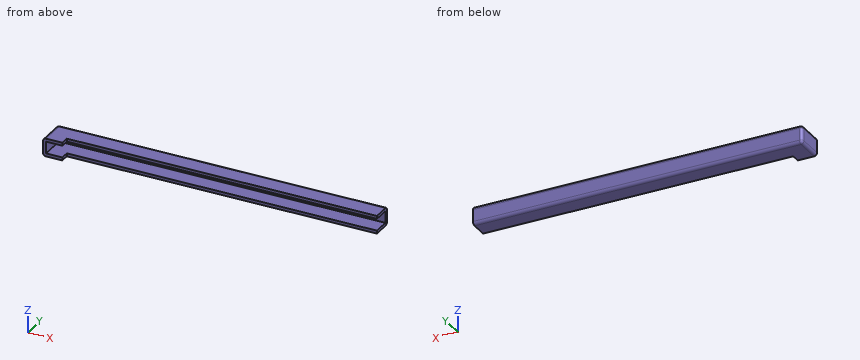
```python
from build123d import *

# Parameters (mm, degrees)
BOSS_EXTRUDE1_DEPTH = 220
SKETCH2_W           = 12
SKETCH2_H           = 13
BOSS_EXTRUDE2_DEPTH = 2
BOSS_EXTRUDE3_DEPTH = 5.8
FILLET1_R           = 2


with BuildPart() as part:
    # Sketch1 → Boss-Extrude1 (new body)
    with BuildSketch(Plane(origin=(0, 0, 0), x_dir=(0, 0, -1), z_dir=(1, 0, 0))):
        Polygon((8, 0), (8, 11), (0, 11), (0, 0), (-2, 0), (-2, 13), (10, 13), (10, 0), align=None)
    extrude(amount=BOSS_EXTRUDE1_DEPTH)

    # Sketch2 → Boss-Extrude2 (add)
    with BuildSketch(Plane.ZY):
        with Locations((-4, 6.5)):
            Rectangle(SKETCH2_W, SKETCH2_H)
    extrude(amount=BOSS_EXTRUDE2_DEPTH)

    # Sketch4 → Boss-Extrude3 (add)
    with BuildSketch(Plane.XZ):
        Polygon((0, 0), (11, 0), (11, 2), (-2, 2), (-2, -10), (11, -10), (11, -8), (0, -8), align=None)
    extrude(amount=BOSS_EXTRUDE3_DEPTH)

    # Fillet1
    fillet1_edges = [part.edges().sort_by_distance(p)[0] for p in [
        (109, 13, 2),
        (109, 13, -10),
        (-2, 3.6, -10),
        (-2, 3.6, 2),
        (-2, 13, -4),
    ]]
    fillet(fillet1_edges, radius=FILLET1_R)


solid = part.part
```
Input: part model. Units: mm. Frame: model coordinates. Coordinates: 2 decimals unless noted, no trailing zeros. Loops run counter-clockwise (first coordinate to the right, second up) from the corner with the lowest first, then second, coordinate; pieces in that order, holes last.
Q1. Section B-B, the plane y = 6.75. Return the cut outline in (x, z).
Results are:
outline: (-2, -8) arc R2 ccw to (0, -10) - (220, -10) - (220, -8) - (0, -8) - (0, 0) - (220, 0) - (220, 2) - (0, 2) arc R2 ccw to (-2, 0) - close
Q2. Section A-A, the plane z = -2.5. Return the cut outline in (x, y).
Results are:
outline: (-2, -5.8) - (0, -5.8) - (0, 11) - (220, 11) - (220, 13) - (0, 13) arc R2 ccw to (-2, 11) - close
Q3. Line query: line 1 along Z through (x, y) = (105, 10.75); line 2 along Y through (x, z) = (124, -3.5); line 3 along X through (y, z) = (0.25, -6.25). Output: solid intervals per line, ascending.
Results are:
line 1: z = -10 to -8, 0 to 2
line 2: y = 11 to 13
line 3: x = -2 to 0
Q4. Contact query for flat-ended pins moving along their axis: pin 1 (4 mm diameter, centred on y = 6, z = -2.5, fed in from +X); pin 2 (5 mm diameter, centred on x = 119.5, z = -4.5, fed in from -Y); pin 3 (0.6 mm diameter, centred on x = 129.5, z = -9, fed in from -Y). Output: stop coordinate, or through.
Results are:
pin 1: stops at x = 0
pin 2: stops at y = 11
pin 3: stops at y = 0
Q5. Section C-C, the plane x = 43. Return the cut outline in (y, z).
Results are:
outline: (0, -10) - (11, -10) arc R2 ccw to (13, -8) - (13, 0) arc R2 ccw to (11, 2) - (0, 2) - (0, 0) - (11, 0) - (11, -8) - (0, -8) - close
